from build123d import *

# Parameters (mm, degrees)
F0_R     = 19.8242320165
F1_DEPTH = 5.08
F0_R_2   = 27.1027644971
F2_DEPTH = 10.16
F4_DEPTH = 25.4


with BuildPart() as f1:
    # F0 (on Top) → F1 (new body)
    with BuildSketch(Plane.XY):
        Circle(F0_R)
    extrude(amount=F1_DEPTH)

    # F0 (on Top) → F2 (join)
    with BuildSketch(Plane.XY):
        Circle(F0_R_2)
        Circle(F0_R, mode=Mode.SUBTRACT)
    extrude(amount=F2_DEPTH)

    # F3 (on face) → F4 (join)
    with BuildSketch(Plane.XY.offset(10.16)):
        with BuildLine():
            ThreePointArc((27.1027644971, 0), (27.0980286069, 0.5066448501), (27.0838225914, 1.0131126398))
            ThreePointArc((27.0838225914, 1.0131126398), (23.0888262615, 3.676897102), (19.823615331, 0.1563657619))
            ThreePointArc((19.823615331, 0.1563657619), (19.8240778445, 0.078183489), (19.8242320165, 0))
            ThreePointArc((19.8242320165, 0), (19.8240778445, -0.078183489), (19.823615331, -0.1563657619))
            ThreePointArc((19.823615331, -0.1563657619), (23.0888262615, -3.676897102), (27.0838225914, -1.0131126398))
            ThreePointArc((27.0838225914, -1.0131126398), (27.0980286069, -0.5066448501), (27.1027644971, 0))
        make_face()
        with BuildLine():
            ThreePointArc((24.0736841586, 11.7613608018), (24.0456154002, 12.2163951196), (23.9618347156, 12.6645300128))
            ThreePointArc((23.9618347156, 12.6645300128), (23.4716825672, 13.5513822485), (22.9487220759, 14.4192925786))
            ThreePointArc((22.9487220759, 14.4192925786), (18.157061535, 14.7286994282), (17.0895715906, 10.0472243876))
            ThreePointArc((17.0895715906, 10.0472243876), (17.1682885368, 9.9121160082), (17.2459373524, 9.7763909435))
            ThreePointArc((17.2459373524, 9.7763909435), (21.404850558, 8.206145204), (24.0736841586, 11.7613608018))
        make_face()
        with BuildLine():
            ThreePointArc((22.9487220759, -14.4192925786), (23.4716825672, -13.5513822485), (23.9618347156, -12.6645300128))
            ThreePointArc((23.9618347156, -12.6645300128), (24.0456154002, -12.2163951196), (24.0736841586, -11.7613608018))
            ThreePointArc((24.0736841586, -11.7613608018), (21.404850558, -8.206145204), (17.2459373524, -9.7763909435))
            ThreePointArc((17.2459373524, -9.7763909435), (17.1682885368, -9.9121160082), (17.0895715906, -10.0472243876))
            ThreePointArc((17.0895715906, -10.0472243876), (18.157061535, -14.7286994282), (22.9487220759, -14.4192925786))
        make_face()
        with BuildLine():
            ThreePointArc((15.4637704856, 20.3712744748), (15.1927300486, 21.7617932839), (14.4192925786, 22.9487220759))
            ThreePointArc((14.4192925786, 22.9487220759), (13.5513822485, 23.4716825672), (12.6645300128, 23.9618347156))
            ThreePointArc((12.6645300128, 23.9618347156), (8.3601268333, 21.833958637), (9.7763909435, 17.2459373524))
            ThreePointArc((9.7763909435, 17.2459373524), (9.9121160082, 17.1682885368), (10.0472243876, 17.0895715906))
            ThreePointArc((10.0472243876, 17.0895715906), (13.6798761402, 17.2047090858), (15.4637704856, 20.3712744748))
        make_face()
        with BuildLine():
            ThreePointArc((12.6645300128, -23.9618347156), (13.5513822485, -23.4716825672), (14.4192925786, -22.9487220759))
            ThreePointArc((14.4192925786, -22.9487220759), (15.1927300486, -21.7617932839), (15.4637704856, -20.3712744748))
            ThreePointArc((15.4637704856, -20.3712744748), (13.6798761402, -17.2047090858), (10.0472243876, -17.0895715906))
            ThreePointArc((10.0472243876, -17.0895715906), (9.9121160082, -17.1682885368), (9.7763909435, -17.2459373524))
            ThreePointArc((9.7763909435, -17.2459373524), (8.3601268333, -21.833958637), (12.6645300128, -23.9618347156))
        make_face()
        with BuildLine():
            ThreePointArc((3.7024096838, 23.5227216035), (2.9545554247, 25.7539633451), (1.0131126398, 27.0838225914))
            ThreePointArc((1.0131126398, 27.0838225914), (0, 27.1027644971), (-1.0131126398, 27.0838225914))
            ThreePointArc((-1.0131126398, 27.0838225914), (-3.676897102, 23.0888262615), (-0.1563657619, 19.823615331))
            ThreePointArc((-0.1563657619, 19.823615331), (0, 19.8242320165), (0.1563657619, 19.823615331))
            ThreePointArc((0.1563657619, 19.823615331), (2.6727109437, 20.9606026215), (3.7024096838, 23.5227216035))
        make_face()
        with BuildLine():
            ThreePointArc((-1.0131126398, -27.0838225914), (0, -27.1027644971), (1.0131126398, -27.0838225914))
            ThreePointArc((1.0131126398, -27.0838225914), (2.9545554247, -25.7539633451), (3.7024096838, -23.5227216035))
            ThreePointArc((3.7024096838, -23.5227216035), (2.6727109437, -20.9606026215), (0.1563657619, -19.823615331))
            ThreePointArc((0.1563657619, -19.823615331), (0, -19.8242320165), (-0.1563657619, -19.823615331))
            ThreePointArc((-0.1563657619, -19.823615331), (-3.676897102, -23.0888262615), (-1.0131126398, -27.0838225914))
        make_face()
        with BuildLine():
            ThreePointArc((-8.0589511179, 20.3712744748), (-9.4849672688, 23.2911837114), (-12.6645300128, 23.9618347156))
            ThreePointArc((-12.6645300128, 23.9618347156), (-13.5513822485, 23.4716825672), (-14.4192925786, 22.9487220759))
            ThreePointArc((-14.4192925786, 22.9487220759), (-14.7286994282, 18.157061535), (-10.0472243876, 17.0895715906))
            ThreePointArc((-10.0472243876, 17.0895715906), (-9.9121160082, 17.1682885368), (-9.7763909435, 17.2459373524))
            ThreePointArc((-9.7763909435, 17.2459373524), (-8.5165950866, 18.5882060743), (-8.0589511179, 20.3712744748))
        make_face()
        with BuildLine():
            ThreePointArc((-14.4192925786, -22.9487220759), (-13.5513822485, -23.4716825672), (-12.6645300128, -23.9618347156))
            ThreePointArc((-12.6645300128, -23.9618347156), (-9.4849672688, -23.2911837114), (-8.0589511179, -20.3712744748))
            ThreePointArc((-8.0589511179, -20.3712744748), (-8.5165950866, -18.5882060743), (-9.7763909435, -17.2459373524))
            ThreePointArc((-9.7763909435, -17.2459373524), (-9.9121160082, -17.1682885368), (-10.0472243876, -17.0895715906))
            ThreePointArc((-10.0472243876, -17.0895715906), (-14.7286994282, -18.157061535), (-14.4192925786, -22.9487220759))
        make_face()
        with BuildLine():
            ThreePointArc((-16.668864791, 11.7613608018), (-18.9281752909, 15.1709505443), (-22.9487220759, 14.4192925786))
            ThreePointArc((-22.9487220759, 14.4192925786), (-23.4716825672, 13.5513822485), (-23.9618347156, 12.6645300128))
            ThreePointArc((-23.9618347156, 12.6645300128), (-21.833958637, 8.3601268333), (-17.2459373524, 9.7763909435))
            ThreePointArc((-17.2459373524, 9.7763909435), (-17.1682885368, 9.9121160082), (-17.0895715906, 10.0472243876))
            ThreePointArc((-17.0895715906, 10.0472243876), (-16.7755794095, 10.8788561477), (-16.668864791, 11.7613608018))
        make_face()
        with BuildLine():
            ThreePointArc((-23.9618347156, -12.6645300128), (-23.4716825672, -13.5513822485), (-22.9487220759, -14.4192925786))
            ThreePointArc((-22.9487220759, -14.4192925786), (-18.9281752909, -15.1709505443), (-16.668864791, -11.7613608018))
            ThreePointArc((-16.668864791, -11.7613608018), (-16.7755794095, -10.8788561477), (-17.0895715906, -10.0472243876))
            ThreePointArc((-17.0895715906, -10.0472243876), (-17.1682885368, -9.9121160082), (-17.2459373524, -9.7763909435))
            ThreePointArc((-17.2459373524, -9.7763909435), (-21.833958637, -8.3601268333), (-23.9618347156, -12.6645300128))
        make_face()
        with BuildLine():
            ThreePointArc((-19.823615331, 0.1563657619), (-23.0888262615, 3.676897102), (-27.0838225914, 1.0131126398))
            ThreePointArc((-27.0838225914, 1.0131126398), (-27.1027644971, 0), (-27.0838225914, -1.0131126398))
            ThreePointArc((-27.0838225914, -1.0131126398), (-23.0888262615, -3.676897102), (-19.823615331, -0.1563657619))
            ThreePointArc((-19.823615331, -0.1563657619), (-19.8242320165, 0), (-19.823615331, 0.1563657619))
        make_face()
    extrude(amount=F4_DEPTH)


solid = f1.part
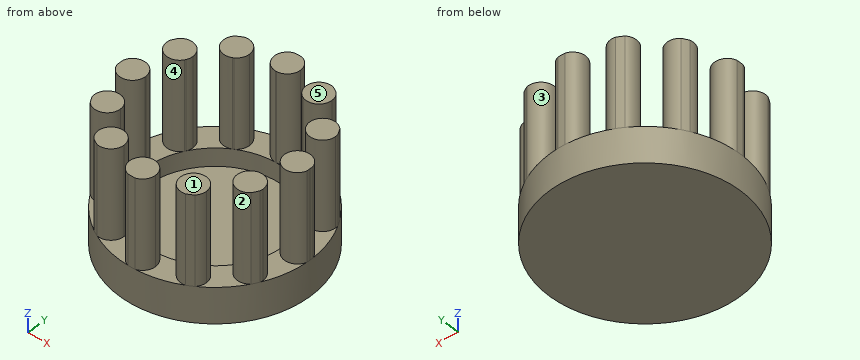
Read the model definition and answer for the solid it produces. Units are mm, in the model's axes. Face numbers are marked on the shaded views. A direction names the side the tool comes from. Give positions to 0.01 mm unless a question says otherwise; leave off trailing zeros. Write each loop counter-clockwise with the first axis right and the second up, starting at its lowest first coordinate (ties: lowest second). Pieces come first, ordered by that corner, then holes. Notation, with made-up numbers: (21.25, -28.75) - (77.25, -28.75) arc R7 ccw to (77.25, -15.75) - close; hole circle Ø11 at (84.5, -11.75). An arc over 180 degrees is marked (long way). Return JSON: item names as keys, results as strings.
Q1. A cutting plane is placed at C-C, the plane x = -21.5. Determine the outline of the cut face in (y, z).
Reply:
{"outline": "(-16.5, 0) - (16.5, 0) - (16.5, 10.16) - (15.29, 10.16) - (15.29, 35.56) - (8.24, 35.56) - (8.24, 10.16) - (3.1, 10.16) - (3.1, 35.56) - (-3.1, 35.56) - (-3.1, 10.16) - (-8.24, 10.16) - (-8.24, 35.56) - (-15.29, 35.56) - (-15.29, 10.16) - (-16.5, 10.16) - close"}
Q2. Given P1, Ø10, axis at y = -14, z = 22.5, coming from the -X side; P2, Ø4, axis at y = -15.5, z = 28, coming from the +X side; P3, Ø3, axis at x = 6, y = -21, coming from the +Z side, each flat-ended and moving along its own axis, determine where each tip first touches the part or whether it passes through.
Reply:
{"P1": "x = -24.07", "P2": "x = 23.5", "P3": "z = 10.16"}
Q3. A cutting plane is placed at B-B, the plane z = 25. Count the separate pieces of the cut face and the enclosed holes in it, and give its area (3 significant figures).
Reply:
{"separate pieces": "12", "enclosed holes": "0", "area": "515 mm²"}
Q4. For the marked faces 1 and 2, determine the directions among +Z, -Z, +X, -X, +Y, -Y from which every point of the face is accessible in a straight line to the end or side of a thin tool.
Reply:
{"face 1": "+Z, +X, -X, +Y, -Y", "face 2": "+Z"}
Q5. For a pull along X with two mould halves and no side action, classify the marked faces 3, 4 and 5 as released by +X, released by -X, zero draft, split by the parting line, or undercut.
Reply:
{"face 3": "undercut", "face 4": "undercut", "face 5": "zero draft"}
Q6. A cutting plane is placed at A-A, the plane x = 5.5. Determine the outline of the cut face in (y, z), and give its area (3 significant figures).
Reply:
{"outline": "(-26.54, 0) - (26.54, 0) - (26.54, 10.16) - (19.05, 10.16) - (19.05, 5.08) - (-19.05, 5.08) - (-19.05, 10.16) - (-26.54, 10.16) - close", "area": "346 mm²"}
Q7. Consider line 1 along Y through (x, z) = (0, 7.9); line 2 along Y through (x, z) = (23, 13.5); line 3 along Y through (x, z) = (12, 34). Determine where each line is inside the solid, lowest interval first. Write a range as [from, to].
Reply:
{"line 1": "[-27.1, -19.82], [19.82, 27.1]", "line 2": "[-14.34, -9.15], [-3.67, 3.67], [9.15, 14.34]", "line 3": "[-24.07, -16.68], [16.68, 24.07]"}
